Work out the finished part from the listing and answer in its coordinate system (mm). Round coordinates to 2 decimals unless told otherwise and drop trailing zeros.
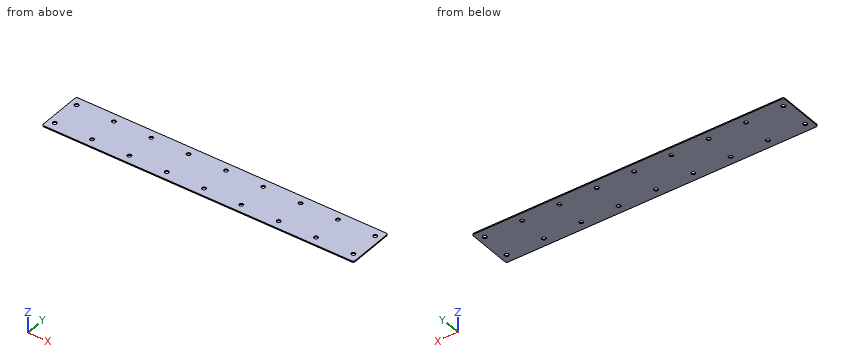
Autodesk Inventor part; units mm, degrees
ref_plane "YZ Plane" through (0, 0, 0) normal (1, 0, 0) x (0, 1, 0)
ref_plane "XZ Plane" through (0, 0, 0) normal (0, 1, 0) x (-1, 0, 0)
ref_plane "XY Plane" through (0, 0, 0) normal (0, 0, 1) x (1, 0, 0)
sketch "Sketch1" plane through (0, 0, 0) normal (0, 0, 1) x (1, 0, 0)
  line L0 (-417.5, 62.5) -> (417.5, 62.5)
  line L1 (417.5, 62.5) -> (417.5, -62.5)
  line L2 (417.5, -62.5) -> (-417.5, -62.5)
  line L3 (-417.5, -62.5) -> (-417.5, 62.5)
  line L4 (-417.5, 62.5) -> (417.5, -62.5) construction
  line L5 (417.5, 62.5) -> (-417.5, -62.5) construction
  point P0 (0, 0)
  dimension "d0" = 125
  dimension "d1" = 835
extrude "Plate1" add sketch "Sketch1" along normal blind 3
sketch "Sketch2" plane through (0, 0, 3) normal (0, 0, 1) x (1, 0, 0)
  circle A0 centre (0, 40) radius 5.35
  circle A1 centre (0, -40) radius 5.35
  line L0 (0, 40) -> (0, -40)
  point P0 (0, 0)
  point P1 (0, 0)
  dimension "d3" = 10.7
  dimension "d4" = 80
extrude "Cut1" cut sketch "Sketch2" against normal blind 3
pattern_linear "Rectangular Pattern1" count 9 spacing 100 along (1, 0, 0) of "Cut1" first direction both ways yes
fillet "Fillet1" radius 5 4 edges at (417.5, -62.5, 1.5) (417.5, 62.5, 1.5) (-417.5, -62.5, 1.5) (-417.5, 62.5, 1.5)
equation "\"d5\" = Thickness"
equation "\"d2\" = Thickness"
equation "\"BendRadius\" = Thickness"
equation "\"BendReliefWidth\" = Thickness"
equation "\"BendReliefDepth\" = 0.5 * Thickness"
equation "\"CornerReliefSize\" = 4 * Thickness"
equation "\"MinimumRemnant\" = 2 * Thickness"
equation "\"TransitionRadius\" = BendRadius"
equation "\"JacobiRadiusSize\" = BendRadius"
equation "\"GapSize\" = Thickness"
properties part number "IMS-10-002" material "Steel, Carbon"
1. Given pin 1 (3 mm diameter, centred on x = 181.5, y = 26.5, fed in from -Z), flat-ended and moving along its own axis, determine where the tip first touches the part or whether it passes through.
Answer key:
pin 1: stops at z = 0
2. Consider probe 1 along Y at (x, z) = (300, 0.9). Determine where the line is inside the solid, lowest interval first.
Answer key:
probe 1: y = -62.5 to -45.35, -34.65 to 34.65, 45.35 to 62.5
3. Find section A-A (z = 1.8). Give the number of separate pieces and of enclosed holes in the cut face, then the cut area to 3 significant figures.
Answer key:
separate pieces: 1
enclosed holes: 18
area: 103,000 mm2
